Part print with two shaded views. Sizes in mm from the minimum x, y, z corner. A direction names the side the tool comes from. Give positions to 0.01 mm unless a question says otherwise; leave off trailing zeros. Return JSON: item names as keys, results as strings. Group by question number.
1. Slice it at A-A on y = 10.16. Give the number of separate pieces and of enclosed holes in the cut face.
2. Wall check: probe 1 along X at (y, z) = (10.75, 19) (1 decimal); probe 2 along X at (y, z) = (10, 12.25) (1 decimal); probe 3 along X at (y, z) = (12, 21.5) (1 decimal). Give the ranges that are in metal, low to high. Write a range as [from, to].
3. 3-axis set-ups, long thin cutter, end or side, ignore diameter. For the marked faces 1 and 2: which of +Z, -Z, +X, -X, +Y, -Y reach the whole face in a straight line?
4. Pin check, flat tips, straight feed: pin 1 (3 mm diameter, centred on x = 27, y = 9.5, fed in from +Z) (1 decimal); pin 2 (7.5 mm diameter, centred on x = 9.5, y = 12.5, fed in from -Z); pin 3 (8 mm diameter, centred on x = 26.99, y = 10.16, fed in from -Z); pin 4 (5 mm diameter, centred on x = 28, y = 12.5, fed in from -Z). Stop position of each tip, or through.
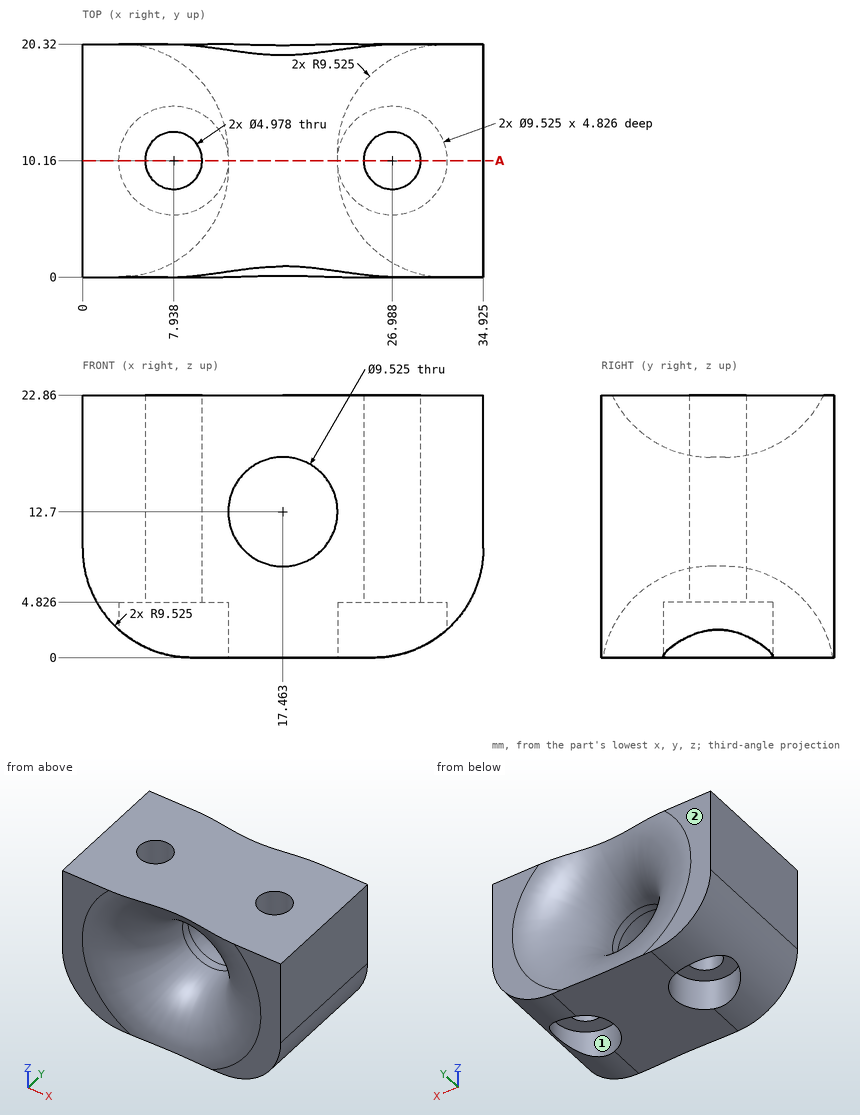
Result:
{
 "1": {"separate pieces": "3", "enclosed holes": "1"},
 "2": {"probe 1": "x = [0, 5.5], [10.4, 24.6], [29.4, 34.9]", "probe 2": "x = [0, 5.5], [10.4, 12.7], [22.2, 24.5], [29.5, 34.9]", "probe 3": "x = [0, 6.3], [9.6, 25.3], [28.7, 34.9]"},
 "3": {"face 1": "-Z", "face 2": "+Z, -Z, +X, -X, +Y"},
 "4": {"pin 1": "passes through", "pin 2": "stops at z = 0", "pin 3": "stops at z = 4.83", "pin 4": "stops at z = 0.2"}
}
